from build123d import *

# Parameters (mm, degrees)
BOSS_EXTRUDE1_DEPTH = 2.54
BOSS_EXTRUDE2_START = -2.54
BOSS_EXTRUDE2_DEPTH = 2.54
CIRPATTERN1_COUNT   = 6
FILLET1_R           = 5.08
FILLET2_R           = 5.08


with BuildPart() as part:
    # Sketch2 → Boss-Extrude1 (new body)
    with BuildSketch(Plane(origin=(0, 0, 0), x_dir=(1, 0, 0), z_dir=(0, 1, 0))):
        with BuildLine():
            Line((110.196456712, 70.954302365), (6.35, 10.998522628))
            Line((6.35, 10.998522628), (6.35, 130.910082102))
            ThreePointArc((6.35, 130.910082102), (0, 131.064), (-6.35, 130.910082102))
            Line((-6.35, 130.910082102), (-6.35, 10.998522628))
            Line((-6.35, 10.998522628), (-110.196456712, 70.954302365))
            ThreePointArc((-110.196456712, 70.954302365), (-113.504753522, 65.532), (-116.546456712, 59.955779737))
            Line((-116.546456712, 59.955779737), (-12.7, 0))
            Line((-12.7, 0), (-116.546456712, -59.955779737))
            ThreePointArc((-116.546456712, -59.955779737), (-113.504753522, -65.532), (-110.196456712, -70.954302365))
            Line((-110.196456712, -70.954302365), (-6.35, -10.998522628))
            Line((-6.35, -10.998522628), (-6.35, -130.910082102))
            ThreePointArc((-6.35, -130.910082102), (0, -131.064), (6.35, -130.910082102))
            Line((6.35, -130.910082102), (6.35, -10.998522628))
            Line((6.35, -10.998522628), (110.196456712, -70.954302365))
            ThreePointArc((110.196456712, -70.954302365), (113.504753522, -65.532), (116.546456712, -59.955779737))
            Line((116.546456712, -59.955779737), (12.7, 0))
            Line((12.7, 0), (116.546456712, 59.955779737))
            ThreePointArc((116.546456712, 59.955779737), (113.504753522, 65.532), (110.196456712, 70.954302365))
        make_face()
    extrude(amount=BOSS_EXTRUDE1_DEPTH)

    # Sketch3 → Boss-Extrude2 (add)
    with BuildSketch(Plane(origin=(0, 2.54, 0), x_dir=(1, 0, 0), z_dir=(0, 1, 0)).offset(BOSS_EXTRUDE2_START)):
        with BuildLine():
            Line((-69.85, 110.899727664), (-69.85, 104.549727664))
            ThreePointArc((-69.85, 104.549727664), (0, 125.736502475), (69.85, 104.549727664))
            Line((69.85, 104.549727664), (69.85, 110.899727664))
            ThreePointArc((69.85, 110.899727664), (0, 131.064), (-69.85, 110.899727664))
        make_face()
    boss_extrude2 = extrude(amount=BOSS_EXTRUDE2_DEPTH)

    # CirPattern1: Boss-Extrude2 ×6 about axis
    cirpattern1_axis = Axis((0, 2.54, 0), (0, -1, 0))
    for i in range(1, CIRPATTERN1_COUNT):
        add(boss_extrude2.rotate(cirpattern1_axis, i * 360 / CIRPATTERN1_COUNT))

    # Fillet1
    fillet1_edges = [part.edges().sort_by_distance(p)[0] for p in [
        (111.927053617, 1.27, -57.288766117),
        (105.577053617, 1.27, -68.287288745),
        (-6.35, 1.27, -125.576054862),
        (6.35, 1.27, -125.576054862),
        (-105.577053617, 1.27, -68.287288745),
        (-111.927053617, 1.27, -57.288766117),
        (-111.927053617, 1.27, 57.288766117),
        (-105.577053617, 1.27, 68.287288745),
        (-6.35, 1.27, 125.576054862),
        (6.35, 1.27, 125.576054862),
        (105.577053617, 1.27, 68.287288745),
        (111.927053617, 1.27, 57.288766117),
    ]]
    fillet(fillet1_edges, radius=FILLET1_R)

    # Fillet2
    fillet2_edges = [part.edges().sort_by_distance(p)[0] for p in [
        (6.35, 1.27, -10.998522628),
        (12.7, 1.27, 0),
        (6.35, 1.27, 10.998522628),
        (-6.35, 1.27, 10.998522628),
        (-12.7, 1.27, 0),
        (-6.35, 1.27, -10.998522628),
    ]]
    fillet(fillet2_edges, radius=FILLET2_R)


solid = part.part
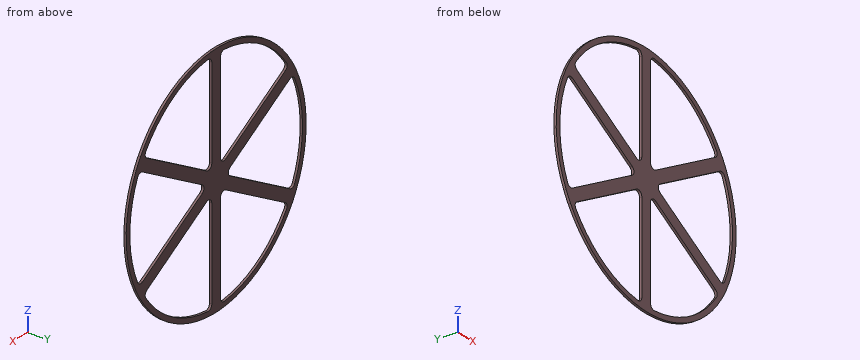
The listing builds one solid part. Answer for the finished solid, in the listing's coordinates (mm). Round coordinates to 2 decimals unless told otherwise and drop trailing zeros. Order: outer loops, then holes, each group sorted by start corner. A loop starts at its lowest first (then second) coordinate and runs counter-clockwise, first axis right, second up. Notation, with made-up numbers: (-39, 28) -> (-18, 28) arc R27 ccw to (-18, 54) -> close; hole circle Ø4 at (19.25, 62). An arc over 180 degrees is marked (long way). Write each question's results on one line, items separated by ' | '. Start each with the question number.
Q1. Find section D-D (y = 1). Give the number of separate pieces and of enclosed holes in the cut face, then the cut area to 3 significant figures.
Q2. Each of these flat-tipped pins is pushed along its axis until it touches: pin 1 (0.8 mm diameter, centred on y = 1, z = -60.5, fed in from +X); pin 2 (1.5 mm diameter, centred on x = -104.5, y = 2, fed in from -Z); pin 3 (1.3 mm diameter, centred on y = 1, z = -76, fed in from -X). Where does it stop, or does it pass through?
Q3. Find section B-B (x = -53.5). Determine the outline of the cut face in (y, z).
Q4. Straight lines are drawn through the part: probe 1 along Z at (x, y) = (-17.5, 1.5); probe 2 along Z at (x, y) = (24, 0.5); probe 3 along Z at (x, y) = (63, 0.6). For each, find the intervals that lie inside material, in ascending order. Write a range as from..to.
Q5. Find section A-A (z = 34). Determine the outline of the cut face in (x, y), then the cut area to 3 significant figures.
Q6. Find section C-C (z = 80.5). Determine the outline of the cut face in (x, y).
Worked answers:
1) separate pieces: 1 | enclosed holes: 6 | area: 13,600 mm2
2) pin 1: stops at x = 116.47 | pin 2: stops at z = -80.09 | pin 3: stops at x = -107.24
3) outline: (0, -119.65) -> (2.54, -119.65) -> (2.54, -113.79) -> (0, -113.79) -> close; (0, -38.22) -> (2.54, -38.22) -> (2.54, -23.56) -> (0, -23.56) -> close; (0, 23.56) -> (2.54, 23.56) -> (2.54, 38.22) -> (0, 38.22) -> close; (0, 113.79) -> (2.54, 113.79) -> (2.54, 119.65) -> (0, 119.65) -> close
4) probe 1: z = -129.89..-124.51, -17.44..17.44, 124.51..129.89 | probe 2: z = -128.85..-123.42, -21.19..-6.52, 6.52..21.19, 123.42..128.85 | probe 3: z = -114.93..-108.81, -43.71..-29.04, 29.04..43.71, 108.81..114.93
5) outline: (-126.58, 0) -> (-121.05, 0) -> (-121.05, 2.54) -> (-126.58, 2.54) -> close; (-71.59, 0) -> (-46.19, 0) -> (-46.19, 2.54) -> (-71.59, 2.54) -> close; (-6.35, 0) -> (6.35, 0) -> (6.35, 2.54) -> (-6.35, 2.54) -> close; (46.19, 0) -> (71.59, 0) -> (71.59, 2.54) -> (46.19, 2.54) -> close; (121.05, 0) -> (126.58, 0) -> (126.58, 2.54) -> (121.05, 2.54) -> close | area: 189 mm2
6) outline: (-103.43, 0) -> (-96.59, 0) -> (-96.59, 2.54) -> (-103.43, 2.54) -> close; (-6.35, 0) -> (6.35, 0) -> (6.35, 2.54) -> (-6.35, 2.54) -> close; (96.59, 0) -> (103.43, 0) -> (103.43, 2.54) -> (96.59, 2.54) -> close
